Input: part model. Units: mm. Frame: model coordinates. Round coordinates to 2 decimals unless told otherwise and drop trailing zeros. Write each loop counter-clockwise with the first axis right and the second up, starting at its lowest first coordinate (ties: lowest second). Pieces come first, ordered by that corner, then holes. Notation, with made-up numbers: (86, -12.75) -> (93, -12.75) arc R26 ccw to (93, 15.25) -> close; hole circle Ø7 at (9, 51.25). An arc over 180 degrees is marked (long way). Use CSV: the item, a comma, the result in double quotes.
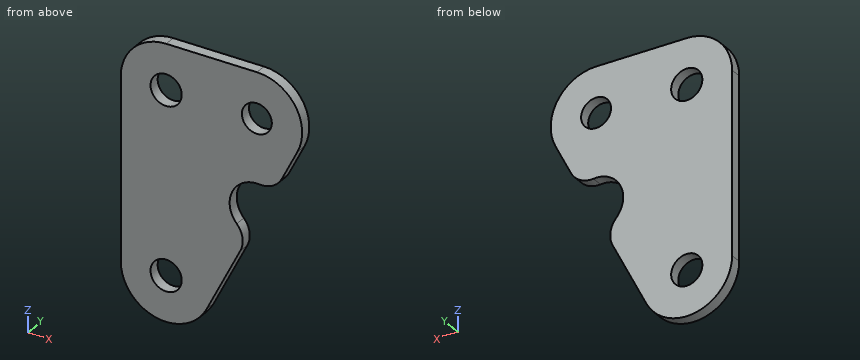
Autodesk Inventor part; units mm, degrees
ref_plane "YZ Plane" through (0, 0, 0) normal (1, 0, 0) x (0, 1, 0)
ref_plane "XZ Plane" through (0, 0, 0) normal (0, 1, 0) x (-1, 0, 0)
ref_plane "XY Plane" through (0, 0, 0) normal (0, 0, 1) x (1, 0, 0)
sketch "Sketch1" plane through (0, 0, 0) normal (0, 1, 0) x (-1, 0, 0)
  circle A0 centre (0, 0) radius 2.1844
  circle A1 centre (0, -25.4) radius 2.1844
  arc A2 (6.35, 0) -> (0, 6.35) centre (0, 0) ccw
  arc A3 (-5.6796, -28.2398) -> (6.35, -25.4) centre (0, -25.4) ccw
  line L0 (6.35, 0) -> (6.35, -25.4)
  circle A4 centre (-12.7, 0) radius 2.0955
  arc A5 (-12.7, 6.35) -> (-18.3796, -2.8398) centre (-12.7, 0) ccw
  line L1 (0, 6.35) -> (-12.7, 6.35)
  arc A6 (-9.8875, -15.2702) -> (-13.0687, -8.9079) centre (-12.7, -12.7) ccw
  line L2 (-18.3796, -2.8398) -> (-16.2157, -7.1677)
  line L3 (-10.3835, -18.8319) -> (-5.6796, -28.2398)
  arc A7 (-9.8875, -15.2702) -> (-10.3835, -18.8319) centre (-7.5437, -17.412) ccw
  arc A8 (-16.2157, -7.1677) -> (-13.0687, -8.9079) centre (-13.3759, -5.7478) ccw
  point P0 (-14.9769, -9.6452)
  point P1 (-11.6223, -16.3544)
  dimension "d0" = 4.3688
  dimension "d1" = 12.7
  dimension "d2" = 4.191
  dimension "d5" = 7.62
  dimension "d6" = 3.175
extrude "Extrusion1" add sketch "Sketch1" along normal blind 1.5875
equation "\"BendRadius\" = Thickness"
equation "\"BendReliefWidth\" = Thickness"
equation "\"BendReliefDepth\" = 0.5 * Thickness"
equation "\"CornerReliefSize\" = 4 * Thickness"
equation "\"MinimumRemnant\" = 2 * Thickness"
equation "\"TransitionRadius\" = BendRadius"
equation "\"JacobiRadiusSize\" = BendRadius"
equation "\"GapSize\" = Thickness"
properties part number "wing_pivot" material "Acetal Resin, White"
Item 1: Section query C-C on x = 7.5. Return the cut outline in (y, z).
Worked answers:
outline,"(0, -24.6) -> (1.59, -24.6) -> (1.59, 6.35) -> (0, 6.35) -> close"
Item 2: First-contact query: pin 1 Ø2 at (x, z) = (-1, -17) entering from -Y. Flat tip, straight axial feed; report the tip coordinate or a pass-through.
Worked answers:
pin 1,"stops at y = 0"
Item 3: Section query B-B on z = -10. Return the cut outline in (x, y).
Worked answers:
outline,"(-6.35, 0) -> (10.01, 0) -> (10.01, 1.59) -> (-6.35, 1.59) -> close"
Item 4: Line query: line 1 (Z direction, x = 0, y = 0.75); line 2 (Z direction, x = -0.75, y = 0.7); line 3 (Z direction, x = 12.7, y = 0.8). Output: solid intervals per line, ascending.
Worked answers:
line 1,"z = -31.75 to -27.58, -23.22 to -2.18, 2.18 to 6.35"
line 2,"z = -31.71 to -27.45, -23.35 to -2.05, 2.05 to 6.31"
line 3,"z = -8.89 to -2.1, 2.1 to 6.35"
Item 5: Section query A-A on y = 0.95. Give the number of separate pieces and of enclosed holes in the cut face, plus the area to 3 significant figures.
Worked answers:
separate pieces,"1"
enclosed holes,"3"
area,"636 mm²"
